Could you check a few things on this model? Use its own coordinates, in mm. A direction names the side the tool comes from. Give positions to 0.01 mm unless a question says otherwise; leave off trailing zeros. Loops run counter-clockwise (first coordinate to the right, second up) from the corner with the lowest first, then second, coordinate; pieces in that order, holes last. Notation, with made-up numbers: (-20, 8) -> (8, 8) arc R20 cw to (8, 47) -> close; hole circle Ø5 at (70, -39.5). An arc over 180 degrees is marked (long way). Put each result on its own line as item: value.
```python
from build123d import *

# Parameters (mm, degrees)
SKETCH1_R               = 48.006
BOSS_EXTRUDE1_DEPTH     = 1.5875
SKETCH2_R               = 46.482
BOSS_EXTRUDE2_DEPTH     = 1.5875
F_1_4_CLEARANCE_HOLE1_D = 6.7564
F_1_4_CLEARANCE_HOLE2_D = 6.7564


with BuildPart() as part:
    # Sketch1 → Boss-Extrude1 (new body, symmetric)
    with BuildSketch(Plane(origin=(0, 0, 0), x_dir=(1, 0, 0), z_dir=(0, 1, 0))):
        Circle(SKETCH1_R)
    extrude(amount=BOSS_EXTRUDE1_DEPTH, both=True)

    # Sketch2 → Boss-Extrude2 (add, symmetric)
    with BuildSketch(Plane(origin=(0, 1.5875, 0), x_dir=(1, 0, 0), z_dir=(0, 1, 0))):
        Circle(SKETCH2_R)
    extrude(amount=BOSS_EXTRUDE2_DEPTH, both=True)

    # 1/4 Clearance Hole1 (through all)
    with Locations(Plane(origin=(0, 3.175, 0), x_dir=(1, 0, 0), z_dir=(0, 1, 0))):
        with Locations((0, 0)):
            Hole(F_1_4_CLEARANCE_HOLE1_D / 2)

    # 1/4 Clearance Hole2 (through all)
    with Locations(Plane(origin=(0, -1.5875, 0), x_dir=(-1, 0, 0), z_dir=(0, -1, 0))):
        with Locations((0, 25.4), (0, -25.4)):
            Hole(F_1_4_CLEARANCE_HOLE2_D / 2)


solid = part.part
```
1. If we section it at C-C (x = 15): List the corners of the cut face in (y, z) for me (1 decimal).
Recorded:
outline: (-1.6, -45.6) -> (1.6, -45.6) -> (1.6, -44) -> (3.2, -44) -> (3.2, 44) -> (1.6, 44) -> (1.6, 45.6) -> (-1.6, 45.6) -> close
2. If we section it at B-B (x = 0): List the corners of the cut face in (y, z) for me (1 decimal).
Recorded:
outline: (-1.6, -48) -> (1.6, -48) -> (1.6, -46.5) -> (3.2, -46.5) -> (3.2, -28.8) -> (-1.6, -28.8) -> close; (-1.6, -22) -> (3.2, -22) -> (3.2, -3.4) -> (-1.6, -3.4) -> close; (-1.6, 3.4) -> (3.2, 3.4) -> (3.2, 22) -> (-1.6, 22) -> close; (-1.6, 28.8) -> (3.2, 28.8) -> (3.2, 46.5) -> (1.6, 46.5) -> (1.6, 48) -> (-1.6, 48) -> close
3. If we section it at A-A (z = 0): List the corners of the cut face in (x, y) for me (1 decimal).
Recorded:
outline: (-48, -1.6) -> (-3.4, -1.6) -> (-3.4, 3.2) -> (-46.5, 3.2) -> (-46.5, 1.6) -> (-48, 1.6) -> close; (3.4, -1.6) -> (48, -1.6) -> (48, 1.6) -> (46.5, 1.6) -> (46.5, 3.2) -> (3.4, 3.2) -> close
4. Thinking about a two-plate mould opening in X: for faces 1 (the face through (21.449, 2.392, 41.238)), 2 (the face through (-0.73, 0.83, -22.1)), 3 (the face through (-1, 3.175, 10)), which applies, pulls with the +X half, pulls with the -X half, needs draft (parallel to the pull), parting line crosses it, or undercut?
Recorded:
face 1: parting line crosses it
face 2: undercut
face 3: needs draft
5. I'm going to push flat-ended pins straight in: pin 1 (2 mm diameter, centred on y = -1, z = 2.5, fed in from +X); pin 2 (9 mm diameter, centred on x = 0, z = 0, fed in from +Y) (3 decimals); pin 3 (2 mm diameter, centred on y = 1.5, z = -31, fed in from -X). Where does each tip first touch, or does it pass through?
Recorded:
pin 1: stops at x = 47.98
pin 2: stops at y = 3.175
pin 3: stops at x = -37.48
6. If we section it at D-D (z = 31.5): List the corners of the cut face in (x, y) for me (1 decimal).
Recorded:
outline: (-36.2, -1.6) -> (36.2, -1.6) -> (36.2, 1.6) -> (34.2, 1.6) -> (34.2, 3.2) -> (-34.2, 3.2) -> (-34.2, 1.6) -> (-36.2, 1.6) -> close
7. For faces 4 (the face through (-10.407, 0.022, 46.864)), 5 (the face through (-25.12, 1.588, -39.34)), which set-ups out of +Z, -Z, +X, -X, +Y, -Y let a thin tool reach every point of the face, with its end or its side?
Recorded:
face 4: +Y, -Y
face 5: +Y
8. I need wall thicknesses on line 1 (Z direction, x = 0, y = 0.7); line 2 (Z direction, x = 2.5, y = 1.7); line 3 (X direction, y = 1.15, z = 25.4). Which ranges of each line are inside material? Lowest first, please.
Recorded:
line 1: z = -48.01 to -28.78, -22.02 to -3.38, 3.38 to 22.02, 28.78 to 48.01
line 2: z = -46.41 to -27.67, -23.13 to -2.27, 2.27 to 23.13, 27.67 to 46.41
line 3: x = -40.74 to -3.38, 3.38 to 40.74
